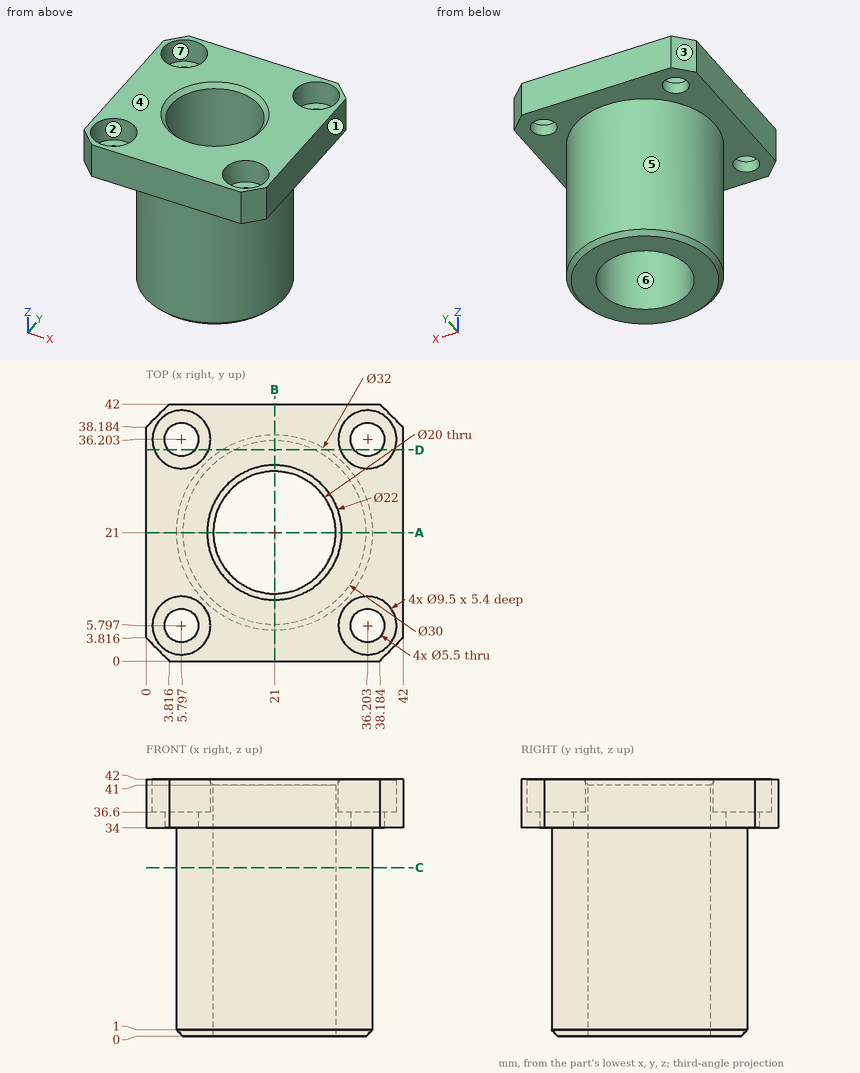
The figure shows three views and two pictorial views of one solid part (mm, origin at its lowest corner). Answer the questions. A direction names the side the tool comes from. Give positions to 0.01 mm unless a question says otherwise; leave off trailing zeros. Loops run counter-clockwise (first coordinate to the right, second up) from the corner with the lowest first, then second, coordinate; pieces in that order, holes last. Notation, with made-up numbers: (-9.75, -23.5) -> (26.25, -23.5) arc R25 ccw to (26.25, -3.5) -> close; hole circle Ø5 at (37.25, -30). An arc over 180 degrees is marked (long way). Use a Markdown table: item, result. Add a question column.
1. Section C-C on z = 27.5 is taken. Determine the outline of the cut face in (x, y), and give its area (3 significant figures).
2. Find the intervals of material crossed by probe 1 along Y at (x, z) = (21, 26); probe 2 along Y at (x, z) = (5.5, 35); probe 3 along Y at (x, z) = (5, 36.5) (1 decimal), in increasing order.
3. For the marked faces 5, 6 and 7, determine the directions among +Z, -Z, +X, -X, +Y, -Y from which every point of the face is accessible in a straight line to the end or side of a thin tool.
4. Flat-ended cylindrical pins translate along their axes: pin 1 Ø10.5 at (x, y) = (4, 7.5) entering from +Z; pin 2 Ø8.5 at (x, y) = (5.8, 36.2) entering from +Z; pin 3 Ø1 at (x, z) = (8.5, 28.5) entering from +Y; pin 4 Ø1.5 at (x, z) = (9, 33) entering from -Y. Find the tip coordinate at first contact, or state that the pin passes through.
5. Determine the mould class of the marked faces 1, 2, 3 and 4 for opening direction X: released by +X, released by -X, zero draft, split by the parting line, or undercut.
6. Section A-A on y = 21 is taken. Determine the outline of the cut face in (x, z), and give its area (3 significant figures).
7. Section D-D on y = 34.5 is taken. State how many separate pieces and enclosed holes the cut face has, and give its area (3 significant figures).
Results below:
| question | item | result |
|---|---|---|
| 1 | outline | circle Ø32 at (21, 21); hole circle Ø20 at (21, 21) |
| 1 | area | 490 mm^2 |
| 2 | probe 1 | y = 5 to 11, 31 to 37 |
| 2 | probe 2 | y = 0 to 3.06, 8.53 to 33.47, 38.94 to 42 |
| 2 | probe 3 | y = 0 to 3.2, 8.4 to 33.6, 38.8 to 42 |
| 3 | face 5 | -Z |
| 3 | face 6 | +Z, -Z |
| 3 | face 7 | +Z |
| 4 | pin 1 | stops at z = 42 |
| 4 | pin 2 | stops at z = 36.6 |
| 4 | pin 3 | stops at y = 31.58 |
| 4 | pin 4 | stops at y = 9.62 |
| 5 | face 1 | released by +X |
| 5 | face 2 | undercut |
| 5 | face 3 | released by -X |
| 5 | face 4 | zero draft |
| 6 | outline | (0, 34) -> (5, 34) -> (5, 1) -> (6, 0) -> (11, 0) -> (11, 41) -> (10, 42) -> (0, 42) -> close; (31, 0) -> (36, 0) -> (37, 1) -> (37, 34) -> (42, 34) -> (42, 42) -> (32, 42) -> (31, 41) -> close |
| 6 | area | 582 mm^2 |
| 7 | separate pieces | 3 |
| 7 | enclosed holes | 0 |
| 7 | area | 800 mm^2 |
